from build123d import *

# Parameters (mm, degrees)
F0_W      = 60
F0_H      = 40
F1_DEPTH  = 50
F2_W      = 20
F2_H      = 10
F3_DEPTH  = 60.001
F5_R      = 35
F6_DEPTH  = 10
F8_DEPTH  = 50.001
F10_DEPTH = 10
F12_DEPTH = 40.001
F14_DEPTH = 40.001


with BuildPart() as f1:
    # F0 (on Top) → F1 (new body)
    with BuildSketch(Plane.XY):
        with Locations((30, 20)):
            Rectangle(F0_W, F0_H)
    extrude(amount=F1_DEPTH)

    # F2 (on face) → F3 (cut, through all)
    with BuildSketch(Plane.YZ.offset(60)):
        with Locations((20, 5)):
            Rectangle(F2_W, F2_H)
    extrude(amount=-F3_DEPTH, mode=Mode.SUBTRACT)

    # F5 (on offset) → F6 (cut)
    with BuildSketch(Plane(origin=(20, 0, 0), x_dir=(0, -1, 0), z_dir=(-1, 0, 0))):
        with Locations((0, 50)):
            Circle(F5_R)
    extrude(amount=F6_DEPTH, mode=Mode.SUBTRACT)

    # F7 (on face) → F8 (cut, through all)
    with BuildSketch(Plane.XY.offset(50)):
        Polygon((40, 0), (60, 0), (60, 30), (45, 20), (30, 0), align=None)
    extrude(amount=-F8_DEPTH, mode=Mode.SUBTRACT)

    # F9 (on face) → F10 (cut, through all)
    with BuildSketch(Plane(origin=(0, 0, 0), x_dir=(0, -1, 0), z_dir=(-1, 0, 0))):
        Polygon((0, 40), (0, 50), (-15, 50), align=None)
    extrude(amount=-F10_DEPTH, mode=Mode.SUBTRACT)

    # F11 (on offset) → F12 (cut, through all)
    with BuildSketch(Plane(origin=(20, 0, 0), x_dir=(0, -1, 0), z_dir=(-1, 0, 0))):
        Polygon((-15, 50), (0, 30), (0, 50), align=None)
    extrude(amount=-F12_DEPTH, mode=Mode.SUBTRACT)

    # F13 (on face) → F14 (cut, through all)
    with BuildSketch(Plane(origin=(0, 40, 0), x_dir=(-1, 0, 0), z_dir=(0, 1, 0))):
        Polygon((-45, 50), (-60, 50), (-60, 10), align=None)
    extrude(amount=-F14_DEPTH, mode=Mode.SUBTRACT)


solid = f1.part
Geometry check sheet. Reference: the model listing, model coordinates, mm. A direction names the side the tool comes from. Give positions to 0.01 mm unless a question says otherwise; leave off trailing zeros. Loops run counter-clockwise (first coordinate to the right, second up) from the corner with the lowest first, then second, coordinate; pieces in that order, holes last.
(1) Section check B-B on y = 21. Record the cut outline in (x, z), then the cut area to 3 significant figures.
From the geometry:
outline: (0, 10) - (46.5, 10) - (46.5, 46) - (45, 50) - (20, 50) - (20, 22) - (10, 22) - (10, 50) - (0, 50) - close
area: 1,580 mm2
(2) Thickness scan on L1, parallel to Y at x = 5.5, z = 8; L2, parallel to X at y = 17, z = 42; L3, parallel to X at y = 10, z = 11.5. Record the ranges inside material, lowest first.
From the geometry:
L1: y = 0 to 10, 30 to 40
L2: x = 0 to 10, 20 to 42.75
L3: x = 0 to 37.5
(3) Section check A-A on z = 4. Record the cut outline in (x, y), then the cut area to 4 significant figures.
From the geometry:
outline: (0, 0) - (30, 0) - (37.5, 10) - (0, 10) - close; (0, 30) - (60, 30) - (60, 40) - (0, 40) - close
area: 937.5 mm2
(4) Section check C-C on x = 17. Record the cut outline in (y, z).
From the geometry:
outline: (0, 0) - (10, 0) - (10, 10) - (30, 10) - (30, 0) - (40, 0) - (40, 50) - (35, 50) arc R35 cw to (0, 15) - close
(5) Release check for a two-part mould opening along X. For faces 1 (the flat face through (15, 0, 11)), 2 (the flat face through (10, 18, 33)), 3 (the flat face through (60, 35, 5)), 4 (the flat face through (0, 20, 25)) record: released by +X, released by -X, zero draft, split by the parting line, or undercut.
From the geometry:
face 1: zero draft
face 2: undercut
face 3: released by +X
face 4: released by -X
(6) Depth check by flat-ended pin: pin 1 Ø6 at (x, y) = (38.5, 20) entering from -Z; pin 2 Ø1 at (x, z) = (16.5, 23.5) entering from -Y; pin 3 Ø1.5 at (x, y) = (12, 24) entering from +Z. Enter the tip coordinate at first touch or a pass-through.
From the geometry:
pin 1: stops at z = 10
pin 2: stops at y = 22.27
pin 3: stops at z = 25.25
(7) Set-up check for faces 5 (the flat face through (49.272, 22.848, 21.391)), 6 (the flat face through (24, 20, 10)), 7 (the flat face through (20, 18, 33)), 8 (the flat face through (28.115, 7.605, 40.14)), 9 (the flat face through (30, 35, 0)): record each of +Z, -Z, +X, -X, +Y, -Y from which the full face is reachable in a straight line by a thin tool's end or side.
From the geometry:
face 5: +Z, -Z, +X, -Y
face 6: -Z, +X, -X
face 7: +Z, -Y
face 8: +Z, +X, -Y
face 9: -Z, +X, -X, +Y, -Y
(8) Section check D-D on z = 17.5. Record the cut outline in (x, y) (1 decimal), then the cut area to 3 significant figures.
From the geometry:
outline: (0, 0) - (10, 0) - (10, 13) - (20, 13) - (20, 0) - (30, 0) - (45, 20) - (57.2, 28.1) - (57.2, 40) - (0, 40) - close
area: 1,710 mm2
